Verification items for the finished model (mm, model axes). Round coordinates to 2 decimals unless told otherwise and drop trailing zeros. Order: outer loops, then holes, each group sorted by start corner. A loop starts at its lowest first (then second) coordinate and runs counter-clockwise, first axis right, second up. Notation, with made-up numbers: M -22.5,-21.5 L -0.5,-21.5 A22 cw -0.5,7.5 Z; hole C -8.75,-30 d2. An arc over 180 degrees is marked long. Use one line per item in the form item = value. Start each with the question number.
Item 1: Cross-section at A-A on z = 2.15. Count the separate pieces of the cut face and the enclosed holes in it, then the cut area to 3 significant figures.
Item 2: Thickness scan on probe 1 along Y at (x, z) = (220.5, 0.2); probe 2 along Y at (x, z) = (213, 1.7); probe 3 along Y at (x, z) = (188, 2.2). Record the ranges inside material, lowest first. Write a range as [from, to].
Item 3: Cross-section at C-C on x = 161.5. Enter the section's corners in (y, z), then the cut area to 3 significant figures.
Item 4: Cross-section at B-B on y = -41.1. Enter the section's corners in (x, z).
Item 5: Cross-section at D-D on x = 174.5. Enter the section's corners in (y, z).
Item 6: Go/stop test with flat-tipped pins: pin 1 Ø2 at (x, z) = (168.5, 1.5) entering from -Y; pin 2 Ø2.5 at (y, z) = (10.5, 2) entering from +X. Record where each tip stops, or that it passes through.
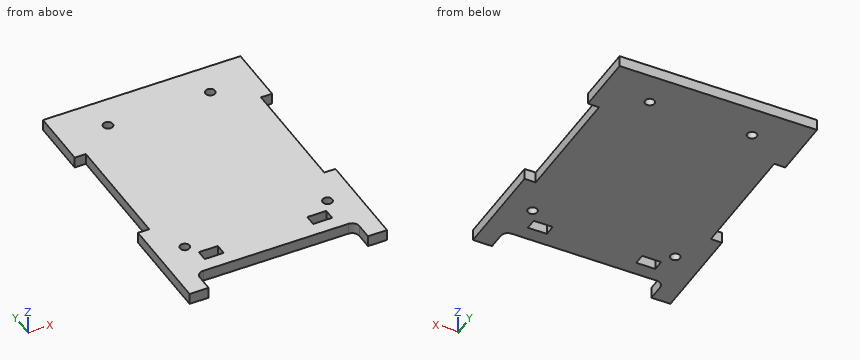
from build123d import *

# Parameters (mm, degrees)
SKETCH013_W             = 8
SKETCH013_H             = 4.7
PAD009_DEPTH            = 4.7
FILLET002_R             = 3
SKETCH020_R             = 2
POCKET002_DEPTH         = 293.388305
BODY015_PLACEMENT_ANGLE = 90


with BuildPart() as part:
    # Sketch013 → Pad009 (new body)
    with BuildSketch(Plane.XZ):
        Polygon((-41.5, -51), (-41.5, -25.5), (-36.8, -25.5), (-36.8, 25.5), (-41.5, 25.5), (-41.5, 51), (41.5, 51), (41.5, 25.5), (36.8, 25.5), (36.8, -25.5), (41.5, -25.5), (41.5, -51), (41.5, -67), (33.5, -67), (33.5, -57), (-33.5, -57), (-33.5, -67), (-41.5, -67), align=None)
        with Locations((-22.8, -48.65)):
            Rectangle(SKETCH013_W, SKETCH013_H, mode=Mode.SUBTRACT)
        with Locations((22.8, -48.65)):
            Rectangle(SKETCH013_W, SKETCH013_H, mode=Mode.SUBTRACT)
    extrude(amount=PAD009_DEPTH)

    # Fillet002
    fillet002_edges = [part.edges().sort_by_distance(p)[0] for p in [
        (-33.5, -2.35, -57),
        (33.5, -2.35, -57),
    ]]
    fillet(fillet002_edges, radius=FILLET002_R)

    # Sketch020 (on Face5 of Fillet002) → Pocket002 (cut, through all)
    with BuildSketch(Plane.XZ.offset(4.7)):
        with Locations((-21.5, 37)):
            Circle(SKETCH020_R)
        with Locations((-30, -41.1)):
            Circle(SKETCH020_R)
    pocket002 = extrude(amount=-POCKET002_DEPTH, mode=Mode.SUBTRACT)

    # Mirrored001: Pocket002 across Sketch020 V_Axis
    add(pocket002.mirror(Plane(origin=(0, -4.7, 0), x_dir=(0, -1, 0), z_dir=(1, 0, 0))), mode=Mode.SUBTRACT)


with BuildPart() as part_1:
    # Body009 placement: moved
    add(part.part.moved(Location((0, -36.8, 48))))


with BuildPart() as part_2:
    # Clone002 placement: moved
    add(part_1.part.moved(Location((0, 36.8, -48))))


with BuildPart() as part_3:
    # Body015 placement: moved
    add(part_2.part.moved(Location((183, 0, 0))).rotate(Axis((183, 0, 0), (-1, 0, 0)), BODY015_PLACEMENT_ANGLE))


solid = part_3.part
Output values:
q1.separate_pieces = 1
q1.enclosed_holes = 6
q1.area = 8,520 mm2
q2.probe_1 = [-67, -25.5], [25.5, 51]
q2.probe_2 = [-57, -43.1], [-39.1, 51]
q2.probe_3 = [-57, 51]
q3.outline = M -57,0 L -51,0 L -51,4.7 L -57,4.7 Z; M -46.3,0 L 35,0 L 35,4.7 L -46.3,4.7 Z; M 39,0 L 51,0 L 51,4.7 L 39,4.7 Z
q3.area = 467 mm2
q4.outline = M 141.5,0 L 151,0 L 151,4.7 L 141.5,4.7 Z; M 155,0 L 211,0 L 211,4.7 L 155,4.7 Z; M 215,0 L 224.5,0 L 224.5,4.7 L 215,4.7 Z
q5.outline = M -57,0 L 51,0 L 51,4.7 L -57,4.7 Z
q6.pin_1 = -57
q6.pin_2 = 219.8
